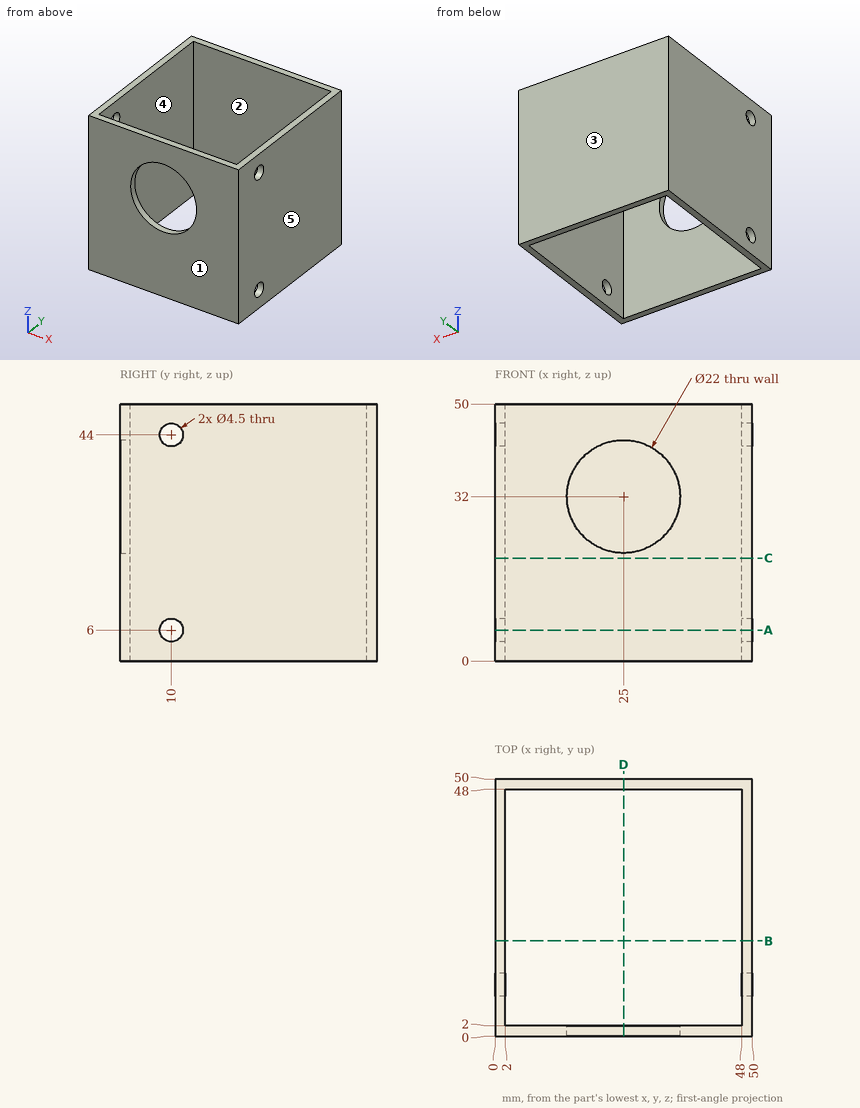
Job drawing, mm, ordinate dimensions from the low corner. One solid piece. A direction names the side the tool comes from. Round coordinates to 2 decimals unless told otherwise and drop trailing zeros. Loops run counter-clockwise (first coordinate to the right, second up) from the corner with the lowest first, then second, coordinate; pieces in that order, holes last.
Item 1: Cut at B-B, the plane y = 18.5. Give the cut face in (x, z).
Item 2: Mould opens along X. For the marked faces 3, 4 and 5 say: +X half, -X half, draft (parallel to the pull), parting line (faces both ways), or undercut.
Item 3: Cut at A-A, the plane z = 6. Give the cut face in (x, y).
Item 4: Cut at C-C, the plane z = 20. Give the cut face in (x, y), then the cut area to 3 significant figures.
Item 5: 3-axis set-ups, long thin cutter, end or side, ignore diameter. For the marked faces 1 and 2: which of +Z, -Z, +X, -X, +Y, -Y reach the whole face in a straight line?
Item 6: Cut at D-D, the plane x = 25. Give the cut face in (y, z), then the cut area to 3 significant figures.
Item 7: Drill centre lines: line 1 (X direction, y = 7, z = 45); line 2 (Z direction, x = 1, y = 10). Where is each one in solid material? Low to high.
A:
1. outline: (0, 0) - (2, 0) - (2, 50) - (0, 50) - close; (48, 0) - (50, 0) - (50, 50) - (48, 50) - close
2. face 3: draft
2. face 4: undercut
2. face 5: +X half
3. outline: (0, 0) - (50, 0) - (50, 7.75) - (48, 7.75) - (48, 2) - (2, 2) - (2, 7.75) - (0, 7.75) - close; (0, 12.25) - (2, 12.25) - (2, 48) - (48, 48) - (48, 12.25) - (50, 12.25) - (50, 50) - (0, 50) - close
4. outline: (0, 0) - (50, 0) - (50, 50) - (0, 50) - close; hole (2, 2) - (48, 2) - (48, 48) - (2, 48) - close
4. area: 384 mm2
5. face 1: +Z, -Z, +X, -X, -Y
5. face 2: +Z, -Z
6. outline: (0, 0) - (2, 0) - (2, 21) - (0, 21) - close; (0, 43) - (2, 43) - (2, 50) - (0, 50) - close; (48, 0) - (50, 0) - (50, 50) - (48, 50) - close
6. area: 156 mm2
7. line 1: x = 0 to 2, 48 to 50
7. line 2: z = 0 to 3.75, 8.25 to 41.75, 46.25 to 50
